```python
from build123d import *

# Parameters (mm, degrees)
CROQUIS1_W                    = 265
CROQUIS1_H                    = 3.175
BRIDA_BASE1_DEPTH             = 25.4
BRIDA_DE_ARISTA1_DEPTH        = 25.4
BRIDA_DE_ARISTA1_BEND_DEPTH   = 25.4
BRIDA_DE_ARISTA2_DEPTH        = 25.4
BRIDA_DE_ARISTA2_BEND_DEPTH   = 25.4
TALADRO_DE_MARGEN_PARA_3_81_D = 10.0838


# Sheet-metal steps are written as plain solids
with BuildPart() as part:
    # Croquis1 → Brida base1 (new body)
    with BuildSketch(Plane.XY):
        with Locations((56.420112782, -1.5875)):
            Rectangle(CROQUIS1_W, CROQUIS1_H)
    extrude(amount=BRIDA_BASE1_DEPTH)

    # Brida de arista1 section (across the edge) → Brida de arista1 (add)
    with BuildSketch(Plane(origin=(189.656712782, -3.175, 0), x_dir=(-1, 0, 0), z_dir=(0, 0, 1))):
        with BuildLine():
            Line((-3.175, 0.7366), (-3.175, 241.825))
            Line((-3.175, 241.825), (0, 241.825))
            Line((0, 241.825), (0, 0.7366))
            ThreePointArc((0, 0.7366), (0.215745145, 0.215745145), (0.7366, 0))
            Line((0.7366, 0), (0.7366, -3.175))
            ThreePointArc((0.7366, -3.175), (-2.029318885, -2.029318885), (-3.175, 0.7366))
        make_face()
    extrude(amount=BRIDA_DE_ARISTA1_DEPTH)

    # Brida de arista1 section 2 (across the edge) → Brida de arista1 bend (add)
    with BuildSketch(Plane(origin=(-76.816487218, -3.175, 25.4), x_dir=(1, 0, 0), z_dir=(0, 0, -1))):
        with BuildLine():
            Line((-3.175, 0.7366), (-3.175, 241.825))
            Line((-3.175, 241.825), (0, 241.825))
            Line((0, 241.825), (0, 0.7366))
            ThreePointArc((0, 0.7366), (0.215745145, 0.215745145), (0.7366, 0))
            Line((0.7366, 0), (0.7366, -3.175))
            ThreePointArc((0.7366, -3.175), (-2.029318885, -2.029318885), (-3.175, 0.7366))
        make_face()
    extrude(amount=BRIDA_DE_ARISTA1_BEND_DEPTH)

    # Brida de arista2 section (across the edge) → Brida de arista2 (add)
    with BuildSketch(Plane(origin=(192.831712782, -245.7366, 25.4), x_dir=(0, 1, 0), z_dir=(0, 0, -1))):
        with BuildLine():
            Line((-3.175, 0.7366), (-3.175, 24.825))
            Line((-3.175, 24.825), (0, 24.825))
            Line((0, 24.825), (0, 0.7366))
            ThreePointArc((0, 0.7366), (0.215745145, 0.215745145), (0.7366, 0))
            Line((0.7366, 0), (0.7366, -3.175))
            ThreePointArc((0.7366, -3.175), (-2.029318885, -2.029318885), (-3.175, 0.7366))
        make_face()
    extrude(amount=BRIDA_DE_ARISTA2_DEPTH)

    # Brida de arista2 section 2 (across the edge) → Brida de arista2 bend (add)
    with BuildSketch(Plane(origin=(-79.991487218, -245.7366, 0), x_dir=(0, 1, 0), z_dir=(0, 0, 1))):
        with BuildLine():
            Line((-3.175, 0.7366), (-3.175, 24.825))
            Line((-3.175, 24.825), (0, 24.825))
            Line((0, 24.825), (0, 0.7366))
            ThreePointArc((0, 0.7366), (0.215745145, 0.215745145), (0.7366, 0))
            Line((0.7366, 0), (0.7366, -3.175))
            ThreePointArc((0.7366, -3.175), (-2.029318885, -2.029318885), (-3.175, 0.7366))
        make_face()
    extrude(amount=BRIDA_DE_ARISTA2_BEND_DEPTH)

    # Taladro de margen para 3/81 (through all)
    with Locations(Plane(origin=(0, -248.9116, 0), x_dir=(-1, 0, 0), z_dir=(0, -1, 0))):
        with Locations((92.816487218, -12.7), (-205.656712782, -12.7)):
            Hole(TALADRO_DE_MARGEN_PARA_3_81_D / 2)


solid = part.part
```
Verification items for the finished model (mm, model axes). A direction names the side the tool comes from. Coordinates: 2 decimals unless noted, no trailing zeros. Order: outer loops, then holes, each group sorted by start corner. A loop starts at its lowest first (then second) coordinate and runs counter-clockwise, first axis right, second up. Notation, with made-up numbers: (32, -16) -> (41, -16) arc R13 ccw to (41, -5) -> close; hole circle Ø10 at (-16.5, 2.25). An arc over 180 degrees is marked (long way). Answer as CSV lines item,"result". Start each with the question number.
1) Set-up check for faces 1 (the face through (-98, -248.912, 13)), 2 (the face through (189.657, -126, 13)), 3 (the face through (200, -245.737, 13)), 4 (the face through (-98, -245.737, 13)): record each of +Z, -Z, +X, -X, +Y, -Y from which the full face is reachable in a straight line by a thin tool's end or side.
2) Cross-section at C-C, the plane x = 96.5. Record the boundary of the cut face in (y, z) (3 decimals), then the cut area to 3 significant figures.
3) Release check for a two-part mould opening along X. For faces 5 (the face through (192.832, -123, 13)), 6 (the face through (-76.816, -126, 13)), 7 (the face through (-79.991, -123, 13)) record: released by +X, released by -X, zero draft, split by the parting line, or undercut.
4) Gauge pin test, flat ends, axial feed: pin 1 Ø7.5 at (y, z) = (-78.5, 11.5) entering from -X; pin 2 Ø11.5 at (x, z) = (205.66, 12.7) entering from +Y; pin 3 Ø4 at (x, z) = (10.5, 16) entering from -Y (3 decimals); pin 4 Ø2 at (x, z) = (-20.5, 23) entering from +Y. Record the tip position at first contact, or that the pin passes through.
5) Cross-section at A-A, the plane z = 12.7. Record the boundary of the cut face in (x, y) (3 decimals).
6) Cross-section at B-B, the plane y = -182. Record the boundary of the cut face in (x, z).
7) Material ranges on L1, parallel to X at y = -208.5, z = 19; L2, parallel to Y at x = 17.5, z = 16 (3 decimals); L3, parallel to Y at x = -86.5, z = 14, recorded low to high. Write a range as [from, to].
Conclusion:
1,face 1,"+Z, -Z, +X, -X, -Y"
1,face 2,"+Z, -Z, -Y"
1,face 3,"+Z, -Z, +X, +Y"
1,face 4,"+Z, -Z, -X, +Y"
2,outline,"(-3.175, 0) -> (0, 0) -> (0, 25.4) -> (-3.175, 25.4) -> close"
2,area,"80.6 mm²"
3,face 5,"released by +X"
3,face 6,"undercut"
3,face 7,"released by -X"
4,pin 1,"stops at x = -79.99"
4,pin 2,"stops at y = -245.74"
4,pin 3,"stops at y = -3.175"
4,pin 4,"stops at y = 0"
5,outline,"(-104.816, -248.912) -> (-97.858, -248.912) -> (-97.858, -245.737) -> (-104.816, -245.737) -> close; (-87.775, -248.912) -> (-80.728, -248.912) arc R3.912 ccw to (-76.816, -245) -> (-76.816, -3.912) arc R0.737 cw to (-76.08, -3.175) -> (188.92, -3.175) arc R0.737 cw to (189.657, -3.912) -> (189.657, -245) arc R3.912 ccw to (193.568, -248.912) -> (200.615, -248.912) -> (200.615, -245.737) -> (193.568, -245.737) arc R0.737 cw to (192.832, -245) -> (192.832, -3.912) arc R3.912 ccw to (188.92, 0) -> (-76.08, 0) arc R3.912 ccw to (-79.991, -3.912) -> (-79.991, -245) arc R0.737 cw to (-80.728, -245.737) -> (-87.775, -245.737) -> close; (210.699, -248.912) -> (217.657, -248.912) -> (217.657, -245.737) -> (210.699, -245.737) -> close"
6,outline,"(-79.99, 0) -> (-76.82, 0) -> (-76.82, 25.4) -> (-79.99, 25.4) -> close; (189.66, 0) -> (192.83, 0) -> (192.83, 25.4) -> (189.66, 25.4) -> close"
7,L1,"x = [-79.99, -76.82], [189.66, 192.83]"
7,L2,"y = [-3.175, 0]"
7,L3,"y = [-248.91, -245.74]"
